Here's how the part is built. I have some questions about the finished solid (model axes, mm). A direction names the side the tool comes from. Give positions to 0.01 mm unless a question says otherwise; leave off trailing zeros. Loops run counter-clockwise (first coordinate to the right, second up) from the corner with the lowest first, then second, coordinate; pieces in that order, holes last. Notation, with made-up numbers: (65.25, 40.25) - (95.25, 40.25) arc R19 cw to (95.25, 53.25) - close; hole circle Ø11 at (52, 83.5). An arc over 180 degrees is marked (long way). Use a Markdown table: item, result.
from build123d import *

# Parameters (mm, degrees)
EXTRUDE_1_DEPTH     = 28
SKETCH_3_R          = 4.25
CUT_EXTRUDE_1_DEPTH = 101.620045975


with BuildPart() as part:
    # 草图1 → 凸台-拉伸1 (new, symmetric)
    with BuildSketch(Plane.XY):
        Polygon((80, 0), (0, 0), (-56.568542495, 56.568542495), (-50.911688245, 62.225396744), (-36.769552622, 48.083261121), (60, 8), (80, 8), align=None)
        with BuildLine():
            Line((52.160622211, 8), (9.638600026, 8))
            Line((9.638600026, 8), (7.747166088, 9.891433938))
            ThreePointArc((7.747166088, 9.891433938), (8.816226337, 12.472373689), (7.747166088, 15.05331344))
            Line((7.747166088, 15.05331344), (6.686505916, 13.992653268))
            ThreePointArc((6.686505916, 13.992653268), (4.343456957, 10.486032694), (5.166226337, 14.622373689))
            Line((5.166226337, 14.622373689), (5.166226337, 16.122373689))
            ThreePointArc((5.166226337, 16.122373689), (2.585286586, 15.05331344), (1.516226337, 12.472373689))
            Line((1.516226337, 12.472373689), (-1.15866519, 12.472373689))
            Line((-1.15866519, 12.472373689), (-31.226275427, 42.539983926))
            Line((-31.226275427, 42.539983926), (52.160622211, 8))
        make_face(mode=Mode.SUBTRACT)
    extrude(amount=EXTRUDE_1_DEPTH, both=True)

    # 草图3 → 切除-拉伸1 (cut, through all)
    with BuildSketch(Plane(origin=(0, 8, 0), x_dir=(1, 0, 0), z_dir=(0, 1, 0))):
        with Locations(Location((70, 0, 0), (0, 0, 180))):
            Circle(SKETCH_3_R)
    cut_extrude_1 = extrude(amount=-CUT_EXTRUDE_1_DEPTH, mode=Mode.SUBTRACT)

    # 镜向1: 切除-拉伸1 across plane
    add(cut_extrude_1.mirror(Plane(origin=(0, 0, 0), x_dir=(0, 0, 1), z_dir=(-0.9238795325112867, 0.3826834323650898, 0))), mode=Mode.SUBTRACT)


solid = part.part
(1) Suppose I cut it at C-C on y = 38.5. Write out the boundary of the cut face in (x, z).
A:
| item | result |
|---|---|
| outline | (-38.5, -28) - (-27.19, -28) - (-27.19, 28) - (-38.5, 28) - close; (-21.47, -28) - (-13.63, -28) - (-13.63, 28) - (-21.47, 28) - close |
(2) Will these pins go through, and if not, where does the flat tip stop? pin 1 (21.5 mm diameter, centred on x = 27, z = 2.5, fed in from +Y); pin 2 (6 mm diameter, centred on y = 15.5, z = 15, fed in from +X); pin 3 (6 mm diameter, centred on x = 74, z = -14, fed in from +Y).
A:
| item | result |
|---|---|
| pin 1 | y = 26.12 |
| pin 2 | x = 49.14 |
| pin 3 | y = 8 |
(3) If I drill on line 1 (Z direction, x = 70, y = 4.5); line 2 (X direction, y = 13.5, z = -18); line 3 (X direction, y = 13, z = -23), over which ranges is the centre line in solid material (lowest first)?
A:
| item | result |
|---|---|
| line 1 | -28 to -4.25, 4.25 to 28 |
| line 2 | -13.5 to -2.19, 1.66 to 3.28, 7.05 to 8.67, 38.88 to 46.72 |
| line 3 | -13 to -1.69, 1.55 to 3.08, 7.25 to 8.78, 40.09 to 47.93 |
(4) Suppose I cut it at D-D on z = -24. Write out the boundary of the cut face in (x, y).
A:
| item | result |
|---|---|
| outline | (-56.57, 56.57) - (0, 0) - (80, 0) - (80, 8) - (60, 8) - (-36.77, 48.08) - (-50.91, 62.23) - close; hole (-31.23, 42.54) - (-1.16, 12.47) - (1.52, 12.47) arc R3.65 cw to (5.17, 16.12) - (5.17, 14.62) arc R2.15 ccw (long way) to (6.69, 13.99) - (7.75, 15.05) arc R3.65 cw to (7.75, 9.89) - (9.64, 8) - (52.16, 8) - close |
(5) Suppose I cut it at B-B on z = 0. Write out the boundary of the cut face in (x, y).
A:
| item | result |
|---|---|
| outline | (-56.57, 56.57) - (-52.5, 52.5) - (-46.85, 58.16) - (-50.91, 62.23) - close; (-46.49, 46.49) - (0, 0) - (65.75, 0) - (65.75, 8) - (60, 8) - (-36.77, 48.08) - (-40.84, 52.15) - close; (74.25, 0) - (80, 0) - (80, 8) - (74.25, 8) - close; hole (-31.23, 42.54) - (-1.16, 12.47) - (1.52, 12.47) arc R3.65 cw to (5.17, 16.12) - (5.17, 14.62) arc R2.15 ccw (long way) to (6.69, 13.99) - (7.75, 15.05) arc R3.65 cw to (7.75, 9.89) - (9.64, 8) - (52.16, 8) - close |
(6) On a 3-axis mill with a long thin cutter (end or side, diameter ignored), from which of +Z, -Z, +X, -X, +Y, -Y can I reach the whole of each face in a straight line? I mean faces 1 (the face through (10.94, 28.32, 0.39)), 2 (the face through (-15.982, 27.296, 0.392)). Say none if no direction works.
A:
| item | result |
|---|---|
| face 1 | +Z, -Z, +X, +Y |
| face 2 | +Z, -Z |
(7) Suppose I cut it at A-A on x = 70. Write out the boundary of the cut face in (y, z), plus the area to 3 significant figures.
A:
| item | result |
|---|---|
| outline | (0, -28) - (8, -28) - (8, -4.25) - (0, -4.25) - close; (0, 4.25) - (8, 4.25) - (8, 28) - (0, 28) - close |
| area | 380 mm2 |
(8) We'd pull the mould along Y, two halves only. Please class faces 3 (the face through (80, 4, 0)), 4 (the face through (65, 8, 0)), 5 (the face through (31, 8, 0)): pulls with the +Y half, pulls with the -Y half, needs draft (parallel to the pull), parting line crosses it, or undercut.
A:
| item | result |
|---|---|
| face 3 | needs draft |
| face 4 | pulls with the +Y half |
| face 5 | undercut |
